Geometry check sheet. Reference: the model listing, model coordinates, mm. A direction names the side the tool comes from. Round coordinates to 2 decimals unless told otherwise and drop trailing zeros. Write each loop counter-clockwise with the first axis right and the second up, starting at its lowest first coordinate (ties: lowest second). Pieces come first, ordered by that corner, then holes.
Item 1: Cross-section at C-C (x = -21.5). Enter the section's corners in (y, z), then the cut area to 3 significant figures.
Item 2: Access from +Z, -Z, +X, -X, +Y, -Y to the whole of each face (thin tool, end or side, straight path). Record for faces 4 (the face through (-53, 7, 16.756)), 5 (the face through (27, 1.2, -8)), 6 (the face through (-11.768, 4, 55)).
Item 3: Depth check by flat-ended pin: P1, Ø0.8, axis at x = -59, z = 37.5, coming from the -Y side; P2, Ø4, axis at y = 4, z = -4, coming from the -X side; P3, Ø3, axis at x = 25.5, z = 15.5, coming from the +Y side. Enter the tip coordinate at first touch or a pass-through.
Item 4: Draft check along X on faces 1 (the face through (-56.912, 0.592, -5.842)), 2 (the face through (6, 4, -2.244)), 3 (the face through (2.232, 4, -6)). Enter one of: pulls with the +X half, pulls with the -X half, needs draft (parallel to the pull), parting line crosses it, or undercut.
Item 5: Scan lines: probe 1 along Z at (x, y) = (-52, 2); probe 2 along Y at (x, z) = (-44, 22); probe 3 along X at (y, z) = (4, 46). Record each from-to range of solid material in increasing order.
Item 6: Cross-section at B-B (z = 5). Enter the section's corners in (x, y).
Item 7: Cross-section at D-D (z = 23.5). Enter the section's corners in (x, y), then the cut area to 3 significant figures.
Item 8: Cross-section at A-A (y = 10.25). Enter the section's corners in (x, z).
from build123d import *

# Parameters (mm, degrees)
SKETCH1_R            = 1.6
PCB_DEPTH            = 1.2
SKETCH2_W            = 6
SKETCH2_H            = 7
POP_CONNECTORS_DEPTH = 4.75
USB_W                = 16
USB_H                = 12.5
USB_B_DEPTH          = 11
SKETCH4_W            = 14.25
SKETCH4_H            = 9.5
DC_POWER_DEPTH       = 11
SKETCH5_W            = 18.982296278
SKETCH5_H            = 16
RJ45_DEPTH           = 13


with BuildPart() as part:
    # Sketch1 → pcb (new body)
    with BuildSketch(Plane(origin=(0, 0, 0), x_dir=(1, 0, 0), z_dir=(0, 1, 0))):
        with BuildLine():
            Line((-54.767524261, 6.744107228), (34.232475739, 6.744107228))
            ThreePointArc((34.232475739, 6.744107228), (36.353796082, 5.865427572), (37.232475739, 3.744107228))
            Line((37.232475739, 3.744107228), (37.232475739, -53.255892772))
            ThreePointArc((37.232475739, -53.255892772), (36.353796082, -55.377213115), (34.232475739, -56.255892772))
            Line((34.232475739, -56.255892772), (-54.767524261, -56.255892772))
            ThreePointArc((-54.767524261, -56.255892772), (-56.888844605, -55.377213115), (-57.767524261, -53.255892772))
            Line((-57.767524261, -53.255892772), (-57.767524261, 3.744107228))
            ThreePointArc((-57.767524261, 3.744107228), (-56.888844605, 5.865427572), (-54.767524261, 6.744107228))
        make_face()
        with Locations((-54.767524261, 3.744107228)):
            Circle(SKETCH1_R, mode=Mode.SUBTRACT)
        with Locations((-54.767524261, -53.255892772)):
            Circle(SKETCH1_R, mode=Mode.SUBTRACT)
        with Locations((34.232475739, -53.255892772)):
            Circle(SKETCH1_R, mode=Mode.SUBTRACT)
        with Locations((34.232475739, 3.744107228)):
            Circle(SKETCH1_R, mode=Mode.SUBTRACT)
    extrude(amount=PCB_DEPTH)

    # Sketch2 → pop connectors (add)
    with BuildSketch(Plane(origin=(0, 1.2, 0), x_dir=(1, 0, 0), z_dir=(0, 1, 0))):
        with Locations((-14.767524261, -55.255892772)):
            Rectangle(SKETCH2_W, SKETCH2_H)
        with Locations((-21.767524261, -55.255892772)):
            Rectangle(SKETCH2_W, SKETCH2_H)
        with Locations((-7.767524261, -55.255892772)):
            Rectangle(SKETCH2_W, SKETCH2_H)
        with Locations((-0.767524261, -55.255892772)):
            Rectangle(SKETCH2_W, SKETCH2_H)
        with Locations((6.232475739, -55.255892772)):
            Rectangle(SKETCH2_W, SKETCH2_H)
        with Locations((13.232475739, -55.255892772)):
            Rectangle(SKETCH2_W, SKETCH2_H)
        with Locations((20.232475739, -55.255892772)):
            Rectangle(SKETCH2_W, SKETCH2_H)
        with Locations((27.232475739, -55.255892772)):
            Rectangle(SKETCH2_W, SKETCH2_H)
        with Locations((27.232475739, 5.744107228)):
            Rectangle(SKETCH2_W, SKETCH2_H)
        with Locations((20.232475739, 5.744107228)):
            Rectangle(SKETCH2_W, SKETCH2_H)
        with Locations((13.232475739, 5.744107228)):
            Rectangle(SKETCH2_W, SKETCH2_H)
        with Locations((6.232475739, 5.744107228)):
            Rectangle(SKETCH2_W, SKETCH2_H)
        with Locations((-0.767524261, 5.744107228)):
            Rectangle(SKETCH2_W, SKETCH2_H)
        with Locations((-7.767524261, 5.744107228)):
            Rectangle(SKETCH2_W, SKETCH2_H)
        with Locations((-14.767524261, 5.744107228)):
            Rectangle(SKETCH2_W, SKETCH2_H)
        with Locations((-21.767524261, 5.744107228)):
            Rectangle(SKETCH2_W, SKETCH2_H)
    extrude(amount=POP_CONNECTORS_DEPTH)

    # usb → USB B (add)
    with BuildSketch(Plane(origin=(0, 1.2, 0), x_dir=(1, 0, 0), z_dir=(0, 1, 0))):
        with Locations((-52.267524261, -7.005892772)):
            Rectangle(USB_W, USB_H)
    extrude(amount=USB_B_DEPTH)

    # Sketch4 → DC power (add)
    with BuildSketch(Plane(origin=(0, 1.2, 0), x_dir=(1, 0, 0), z_dir=(0, 1, 0))):
        with Locations((-53.142524261, -21.505892772)):
            Rectangle(SKETCH4_W, SKETCH4_H)
    extrude(amount=DC_POWER_DEPTH)

    # Sketch5 → RJ45 (add)
    with BuildSketch(Plane(origin=(0, 1.2, 0), x_dir=(1, 0, 0), z_dir=(0, 1, 0))):
        with Locations((-50.776376122, -41.255892772)):
            Rectangle(SKETCH5_W, SKETCH5_H)
    extrude(amount=RJ45_DEPTH)


solid = part.part
Resolved:
1. outline: (0, -6.74) - (1.2, -6.74) - (1.2, -9.24) - (5.95, -9.24) - (5.95, -2.24) - (1.2, -2.24) - (1.2, 51.76) - (5.95, 51.76) - (5.95, 58.76) - (1.2, 58.76) - (1.2, 56.26) - (0, 56.26) - close
1. area: 142 mm2
2. face 4: +X, -X, +Y
2. face 5: -Z, +X, -X, -Y
2. face 6: +Z, -Z, +Y
3. P1: stops at y = 1.2
3. P2: stops at x = -24.77
3. P3: stops at y = 1.2
4. face 1: pulls with the -X half
4. face 2: needs draft
4. face 3: undercut
5. probe 1: z = 0.76 to 13.26, 16.76 to 26.26, 33.26 to 49.26
5. probe 2: y = 0 to 1.2
5. probe 3: x = -60.27 to -41.29
6. outline: (-60.27, 1.2) - (-57.77, 1.2) - (-57.77, 0) - (37.23, 0) - (37.23, 1.2) - (-44.27, 1.2) - (-44.27, 12.2) - (-60.27, 12.2) - close
7. outline: (-60.27, 1.2) - (-57.77, 1.2) - (-57.77, 0) - (37.23, 0) - (37.23, 1.2) - (-46.02, 1.2) - (-46.02, 12.2) - (-60.27, 12.2) - close
7. area: 271 mm2
8. outline: (-60.27, 0.76) - (-44.27, 0.76) - (-44.27, 13.26) - (-60.27, 13.26) - close; (-60.27, 16.76) - (-46.02, 16.76) - (-46.02, 26.26) - (-60.27, 26.26) - close; (-60.27, 33.26) - (-41.29, 33.26) - (-41.29, 49.26) - (-60.27, 49.26) - close
